```python
from build123d import *

# Parameters (mm, degrees)
F1_DEPTH = 25
F2_R     = 10
F3_R     = 2
F4_DEPTH = 12.5
F5_SIZE  = 5
F6_DEPTH = 10
F7_START = -4.5
F3_R_2   = 4.25
F7_DEPTH = 0.9
F8_START = 4.5
F8_DEPTH = 0.9
F9_SIZE  = 0.6
F10_R    = 10


with BuildPart() as f1:
    # F0 (on Top) → F1 (new body)
    with BuildSketch(Plane.XY):
        with BuildLine():
            Line((5.4, 12), (-5.4, 12))
            Line((-5.4, 12), (-5.4, 2))
            Line((-5.4, 2), (-5.4, -2))
            Line((-5.4, -2), (-5.4, -8.0747857195))
            ThreePointArc((-5.4, -8.0747857195), (0, -19.4), (5.4, -8.0747857195))
            Line((5.4, -8.0747857195), (5.4, -2))
            Line((5.4, -2), (5.4, 2))
            Line((5.4, 2), (5.4, 12))
        make_face()
        with BuildLine():
            ThreePointArc((4.45, -12.45), (-2.8692333471, -15.8514702703), (-0.75, -8.0636575601))
            Line((-0.75, -8.0636575601), (-0.75, -8))
            Line((-0.75, -8), (0, -8))
            Line((0, -8), (0.75, -8))
            Line((0.75, -8), (0.75, -8.0636575601))
            ThreePointArc((0.75, -8.0636575601), (3.4014702703, -9.5807666529), (4.45, -12.45))
        make_face(mode=Mode.SUBTRACT)
        with BuildLine():
            ThreePointArc((0.75, -9.5969314765), (0, -15.4), (-0.75, -9.5969314765))
            Line((-0.75, -9.5969314765), (-0.75, -8.0636575601))
            ThreePointArc((-0.75, -8.0636575601), (-2.8692333471, -15.8514702703), (4.45, -12.45))
            ThreePointArc((4.45, -12.45), (3.4014702703, -9.5807666529), (0.75, -8.0636575601))
            Line((0.75, -8.0636575601), (0.75, -9.5969314765))
        make_face()
    extrude(amount=F1_DEPTH)

    # F2
    f2_edges = [f1.edges().sort_by_distance(p)[0] for p in [
        (0, 12, 25),
    ]]
    fillet(f2_edges, radius=F2_R)

    # F3 (on Right) → F4 (cut, symmetric)
    with BuildSketch(Plane.YZ):
        with Locations((0, 12.5)):
            Circle(F3_R)
    extrude(amount=F4_DEPTH, both=True, mode=Mode.SUBTRACT)

    # F5
    f5_edges = [f1.edges().sort_by_distance(p)[0] for p in [
        (0, 12, 0),
    ]]
    chamfer(f5_edges, length=F5_SIZE)

    # F0 (on Top) → F6 (cut)
    with BuildSketch(Plane.XY):
        with BuildLine():
            ThreePointArc((0.75, -9.5969314765), (0, -15.4), (-0.75, -9.5969314765))
            Line((-0.75, -9.5969314765), (-0.75, -8.0636575601))
            ThreePointArc((-0.75, -8.0636575601), (-2.8692333471, -15.8514702703), (4.45, -12.45))
            ThreePointArc((4.45, -12.45), (3.4014702703, -9.5807666529), (0.75, -8.0636575601))
            Line((0.75, -8.0636575601), (0.75, -9.5969314765))
        make_face()
    extrude(amount=F6_DEPTH, mode=Mode.SUBTRACT)

    # F3 (on Right) → F7 (cut)
    with BuildSketch(Plane.YZ.offset(F7_START)):
        with Locations((0, 12.5)):
            Circle(F3_R_2)
        with Locations((0, 12.5)):
            Circle(F3_R, mode=Mode.SUBTRACT)
    extrude(amount=-F7_DEPTH, mode=Mode.SUBTRACT)

    # F3 (on Right) → F8 (cut)
    with BuildSketch(Plane.YZ.offset(F8_START)):
        with Locations((0, 12.5)):
            Circle(F3_R_2)
        with Locations((0, 12.5)):
            Circle(F3_R, mode=Mode.SUBTRACT)
    extrude(amount=F8_DEPTH, mode=Mode.SUBTRACT)

    # F9
    f9_edges = [f1.edges().sort_by_distance(p)[0] for p in [
        (4.5, -4.25, 12.5),
        (-4.5, -4.25, 12.5),
    ]]
    chamfer(f9_edges, length=F9_SIZE)

    # F10
    f10_edges = [f1.edges().sort_by_distance(p)[0] for p in [
        (0, 12, 5),
    ]]
    fillet(f10_edges, radius=F10_R)


solid = f1.part
```
Input: part model. Units: mm. Frame: model coordinates. A direction names the side the tool comes from. Give positions to 0.01 mm unless a question says otherwise; leave off trailing zeros. Write each loop counter-clockwise with the first axis right and the second up, starting at its lowest first coordinate (ties: lowest second). Pieces come first, ordered by that corner, then holes. Notation, with made-up numbers: (49, 77) - (82, 77) arc R24 ccw to (82, 116) - close; hole circle Ø2 at (25, 5.5). An arc over 180 degrees is marked (long way). Write item = value, one per line. Start each with the question number.
1. Section query B-B, the plane z = 12.5. Output: boundary loops of the cut face in (x, y).
2. Ray query, L1, parallel to X at y = -12.45, z = 17.25; L2, parallel to Z at x = 5.3, y = 0; L3, parallel to Z at x = -3.25, y = -12.5. Return the intervals inside material, ascending.
3. Section query A-A, the plane x = 0. Output: boundary loops of the cut face in (y, z), then the cut area to 3 significant figures.
4. Mould query, pull axis Y, two halves, no side actions, for faces 4 (the cylindrical face through (0.1, -15.4, 17.4)), 5 (the flat face through (0, 12, 12)), 6 (the flat face through (-5.4, 4, 10)). Classes: released by +Y, released by -Y, zero draft, split by the parting line, or undercut.
5. Section query D-D, the plane z = 23. Output: boundary loops of the cut face in (x, y).
6. Section query C-C, the plane y = 0. Output: boundary loops of the cut face in (x, z).
7. First-contact query: pin 1 Ø6 at (x, z) = (-2.5, 8.5) entering from -Y; pin 2 Ø2 at (x, z) = (-5, 19.5) entering from +Y; pin 3 Ø0.5 at (y, z) = (-9, 8.5) entering from +X; pin 4 Ø4 at (x, z) = (0, 21) entering from +Y. Flat tips, straight axial feed; report the tip coordinate or a pass-through.
8. Access query for faces 1 (the flat face through (0.75, -9, 18)), 2 (the flat face through (4.5, 2, 11)), 3 (the cylindrical face through (-5.25, -0.92, 8.35)). Directions: +Z, -Z, +X, -X, +Y, -Y. A direction counts if a zero-diameter tool reaches every point of the face in a straight line with its end or side. Return the directions, or none.
Check sheet entries:
q1.outline = (-5.4, -8.07) arc R6.95 ccw (long way) to (5.4, -8.07) - (5.4, -4.25) - (5.1, -4.25) - (4.5, -3.65) - (4.5, -2) - (-4.5, -2) - (-4.5, -3.65) - (-5.1, -4.25) - (-5.4, -4.25) - close; (-5.4, 4.25) - (-5.1, 4.25) - (-4.5, 3.65) - (-4.5, 2) - (4.5, 2) - (4.5, 3.65) - (5.1, 4.25) - (5.4, 4.25) - (5.4, 12) - (-5.4, 12) - close; hole (-0.75, -9.6) arc R2.95 ccw (long way) to (0.75, -9.6) - (0.75, -8) - (-0.75, -8) - close
q2.L1 = -6.95 to -2.95, 2.95 to 6.95
q2.L2 = 0 to 8.25, 16.75 to 25
q2.L3 = 10 to 25
q3.outline = (-19.4, 0) - (-16.9, 0) - (-16.9, 10) - (-15.4, 10) - (-15.4, 25) - (-19.4, 25) - close; (-8, 0) - (7, 0) - (9.07, 2.07) arc R10 ccw to (12, 9.14) - (12, 15) arc R10 ccw to (2, 25) - (-8, 25) - close; hole circle Ø4 at (0, 12.5)
q3.area = 536 mm2
q4.face_4 = undercut
q4.face_5 = released by +Y
q4.face_6 = zero draft
q5.outline = (-5.4, -8.07) arc R6.95 ccw (long way) to (5.4, -8.07) - (5.4, 8) - (-5.4, 8) - close; hole (-0.75, -9.6) arc R2.95 ccw (long way) to (0.75, -9.6) - (0.75, -8) - (-0.75, -8) - close
q6.outline = (-5.4, 0) - (5.4, 0) - (5.4, 8.25) - (5.1, 8.25) - (4.5, 8.85) - (4.5, 10.5) - (-4.5, 10.5) - (-4.5, 8.85) - (-5.1, 8.25) - (-5.4, 8.25) - close; (-5.4, 16.75) - (-5.1, 16.75) - (-4.5, 16.15) - (-4.5, 14.5) - (4.5, 14.5) - (4.5, 16.15) - (5.1, 16.75) - (5.4, 16.75) - (5.4, 25) - (-5.4, 25) - close
q7.pin_1 = -19.4
q7.pin_2 = 11.37
q7.pin_3 = 6.17
q7.pin_4 = 11.17
q8.face_1 = +Z, -Z
q8.face_2 = +X
q8.face_3 = -X
